from build123d import *

# Parameters (mm, degrees)
SKETCH1_R               = 52.5
BOSS_EXTRUDE1_DEPTH     = 10
SKETCH3_R               = 3
CUT_EXTRUDE1_DEPTH      = 75.916620319
SKETCH4_W               = 34.98571137
SKETCH4_H               = 10
SKETCH4_W_2             = 10
SKETCH4_H_2             = 34.98571137
CUT_EXTRUDE_THIN1_DEPTH = 75.916620319
CUT_EXTRUDE3_REACH      = 113.136
CUT_EXTRUDE3_END_RADIUS = 3
SKETCH5_R               = 1.5
CIRPATTERN1_COUNT       = 4
SKETCH6_R               = 12.5
CUT_EXTRUDE4_DEPTH      = 71.714213718
SKETCH7_R               = 1.5
CUT_EXTRUDE5_DEPTH      = 71.714213718


with BuildPart() as part:
    # Sketch1 → Boss-Extrude1 (new body)
    with BuildSketch(Plane(origin=(0, 0, 0), x_dir=(1, 0, 0), z_dir=(0, 1, 0))):
        with Locations(Location((0, 0, 0), (0, 0, 270))):
            Circle(SKETCH1_R)
    extrude(amount=BOSS_EXTRUDE1_DEPTH)

    # Sketch3 → Cut-Extrude1 (cut, through all)
    with BuildSketch(Plane(origin=(0, 10, 0), x_dir=(1, 0, 0), z_dir=(0, 1, 0))):
        with Locations(Location((0, 45, 0), (0, 0, 270))):
            Circle(SKETCH3_R)
        with Locations(Location((45, 0, 0), (0, 0, 270))):
            Circle(SKETCH3_R)
        with Locations(Location((0, -45, 0), (0, 0, 270))):
            Circle(SKETCH3_R)
        with Locations(Location((-45, 0, 0), (0, 0, 270))):
            Circle(SKETCH3_R)
    extrude(amount=-CUT_EXTRUDE1_DEPTH, mode=Mode.SUBTRACT)

    # Sketch4 → Cut-Extrude-Thin1 (cut, through all)
    with BuildSketch(Plane(origin=(0, 10, 0), x_dir=(1, 0, 0), z_dir=(0, 1, 0))):
        with Locations((0, -54.5)):
            Rectangle(SKETCH4_W, SKETCH4_H)
        with Locations((54.5, 0)):
            Rectangle(SKETCH4_W_2, SKETCH4_H_2)
        with Locations((0, 54.5)):
            Rectangle(SKETCH4_W, SKETCH4_H)
        with Locations((-54.5, 0)):
            Rectangle(SKETCH4_W_2, SKETCH4_H_2)
    extrude(amount=-CUT_EXTRUDE_THIN1_DEPTH, mode=Mode.SUBTRACT)

    # Cut-Extrude3: up to this cylinder (the profile starts outside it)
    cut_extrude3_end = Plane(origin=(0, 5, 45), z_dir=(0, 1, 0)) * Cylinder(CUT_EXTRUDE3_END_RADIUS, 233.272, mode=Mode.PRIVATE)
    # Sketch5 → Cut-Extrude3 (cut, up to the surface)
    with BuildSketch(Plane.XY.offset(49.5), mode=Mode.PRIVATE) as cut_extrude3_sk1:
        with Locations((0, 5)):
            Circle(SKETCH5_R)
    cut_extrude3_tool1 = extrude(cut_extrude3_sk1.sketch, amount=-CUT_EXTRUDE3_REACH, mode=Mode.PRIVATE) - cut_extrude3_end
    cut_extrude3 = cut_extrude3_tool1.solids().sort_by_distance((0, 5, 49.5))[0]
    add(cut_extrude3, mode=Mode.SUBTRACT)

    # CirPattern1: Cut-Extrude3 ×4 about axis
    cirpattern1_axis = Axis((0, 10, 0), (0, -1, 0))
    for i in range(1, CIRPATTERN1_COUNT):
        add(cut_extrude3.rotate(cirpattern1_axis, i * 360 / CIRPATTERN1_COUNT), mode=Mode.SUBTRACT)

    # Sketch6 → Cut-Extrude4 (cut, through all)
    with BuildSketch(Plane(origin=(0, 10, 0), x_dir=(1, 0, 0), z_dir=(0, 1, 0))):
        with Locations(Location((0, 0, 0), (0, 0, 270))):
            Circle(SKETCH6_R)
    extrude(amount=-CUT_EXTRUDE4_DEPTH, mode=Mode.SUBTRACT)

    # Sketch7 → Cut-Extrude5 (cut, through all)
    with BuildSketch(Plane(origin=(0, 10, 0), x_dir=(1, 0, 0), z_dir=(0, 1, 0))):
        with Locations(Location((-15.5, 15.5, 0), (0, 0, 270))):
            Circle(SKETCH7_R)
        with Locations(Location((15.5, 15.5, 0), (0, 0, 90))):
            Circle(SKETCH7_R)
        with Locations(Location((15.5, -15.5, 0), (0, 0, 270))):
            Circle(SKETCH7_R)
        with Locations(Location((-15.5, -15.5, 0), (0, 0, 90))):
            Circle(SKETCH7_R)
    extrude(amount=-CUT_EXTRUDE5_DEPTH, mode=Mode.SUBTRACT)


solid = part.part
The model under review builds one solid part; all positions refer to its coordinate system, in mm. A direction names the side the tool comes from. Give positions to 0.01 mm unless a question says otherwise; leave off trailing zeros. Loops run counter-clockwise (first coordinate to the right, second up) from the corner with the lowest first, then second, coordinate; pieces in that order, holes last. Notation, with made-up numbers: (20, 82) -> (43, 82) arc R25 cw to (43, 102) -> close; hole circle Ø8 at (-30.5, 35.25). An arc over 180 degrees is marked (long way). Put each result on its own line as item: value. Start each with the question number.
1. We need section A-A on z = -15.5. State the section outline as (x, y) points.
2. We need section B-B on z = 0. State the section outline as (x, y) points, then the cut area to 3 significant figures.
3. For faces 1 (the face through (-1.43, 5.45, -48.56)), 2 (the face through (-48.56, 5.45, 1.43)), 3 (the face through (1.43, 5.45, 48.56)), list the 3-axis set-ups (+Z, -Z, +X, -X, +Y, -Y) from which the entire face can be reached by the end or side of a thin tool; tool diameter is ignored.
4. Wall thickness on probe 1 along X at (y, z) = (6, 15.5); probe 2 along Y at (x, z) = (-49, 0); probe 3 along Z at (x, y) = (44, 7.25): over which ranges is each line inside the solid? List them lowest first.
5. We need section C-C on x = 45. State the section outline as (y, z) points.
6. We need section D-D on z = 45. State the section outline as (x, y) points.
7. Clearance check with flat-ended pins moving along their axes: P1, Ø1.8, axis at y = 5, z = 0, coming from the +X side; P2, Ø5, axis at y = 1, z = -27.5, coming from the +X side; P3, Ø5, axis at x = -27.5, y = 5.5, coming from the +Z side. State where each tip first meets the part, or that it passes through.
8. Mouldability with a two-part tool opening along X and no side actions: class faces 4 (the face through (-36.891, 4.93, -37.354)), 5 (the face through (37.354, 4.93, -36.891)), 6 (the face through (15.43, 5.07, -14)) as released by +X, released by -X, zero draft, split by the parting line, or undercut.
Determined:
1. outline: (-49.5, 0) -> (-17, 0) -> (-17, 10) -> (-49.5, 10) -> close; (-14, 0) -> (14, 0) -> (14, 10) -> (-14, 10) -> close; (17, 0) -> (49.5, 0) -> (49.5, 10) -> (17, 10) -> close
2. outline: (-49.5, 0) -> (-48, 0) -> (-48, 3.5) -> (-49.5, 3.5) -> close; (-49.5, 6.5) -> (-48, 6.5) -> (-48, 10) -> (-49.5, 10) -> close; (-42, 0) -> (-12.5, 0) -> (-12.5, 10) -> (-42, 10) -> close; (12.5, 0) -> (42, 0) -> (42, 10) -> (12.5, 10) -> close; (48, 0) -> (49.5, 0) -> (49.5, 3.5) -> (48, 3.5) -> close; (48, 6.5) -> (49.5, 6.5) -> (49.5, 10) -> (48, 10) -> close
2. area: 611 mm^2
3. face 1: -Z
3. face 2: -X
3. face 3: +Z
4. probe 1: -49.5 to -17, -14 to 14, 17 to 49.5
4. probe 2: 0 to 3.5, 6.5 to 10
4. probe 3: -28.64 to -2.83, 2.83 to 28.64
5. outline: (0, -27.04) -> (10, -27.04) -> (10, -3) -> (0, -3) -> close; (0, 3) -> (10, 3) -> (10, 27.04) -> (0, 27.04) -> close
6. outline: (-27.04, 0) -> (-3, 0) -> (-3, 10) -> (-27.04, 10) -> close; (3, 0) -> (27.04, 0) -> (27.04, 10) -> (3, 10) -> close
7. P1: x = 42.14
7. P2: x = 46.17
7. P3: z = 46.17
8. face 4: released by -X
8. face 5: released by +X
8. face 6: undercut
